For this review, take the finished solid that the model builds, in its own axes (mm). Face numbers are marked on the shaded views. A direction names the side the tool comes from. Give positions to 0.01 mm unless a question says otherwise; leave off trailing zeros. Write each loop counter-clockwise with the first axis right and the second up, starting at its lowest first coordinate (ties: lowest second). Pieces come first, ordered by that corner, then holes.
Q1. Machinability: for the marked faces 4, 5, 6 and 7, which of the approach directions +Z, -Z, +X, -X, +Y, -Y give a long, thin tool a straight path to every point of the face, cutting with its end or side? Answer none if there is none.
Q2. For line 1 (Z direction, x = 0, y = 9.75); line 2 (Z direction, x = 0.5, y = 4.75); line 3 (X direction, y = 13, z = -5), list the stretches that pass through material, from the lowest coordinate up.
Q3. We need section A-A (y = 5.5). Write out the cut boundary in (x, z) (1 decimal).
Q4. Mouldability with a two-part tool opening along Y and no side actions: class the marked faces 1, 2 and 3 as released by +Y, released by -Y, zero draft, split by the parting line, or undercut.
Q5. We need section B-B (z = -10). Give the number of separate pieces and of enclosed holes in the cut face, then the cut area to 3 significant figures.
Q6. Insertion check: P1, Ø1, axis at y = 9.5, z = -12.5, coming from the +X side; P2, Ø1, axis at x = -4, y = 8, coming from the +Z side; P3, Ø3, axis at y = 8, z = -14, coming from the +X side. Each pin has a flat end and moves straight along its axis. Give the tip position at first contact, or say it passes through.
```python
from build123d import *

# Parameters (mm, degrees)
CUT_EXTRUDE2_DEPTH       = 15.16264375
SKETCH5_W                = 4.35
SKETCH5_H                = 6.35
SKETCH6_R                = 1.5875
BOSS_EXTRUDE2_DEPTH      = 1
BOSS_EXTRUDE2_DEPTH_BACK = 9.525


with BuildPart() as part:
    # Sketch2 → Revolve-Thin1 (revolve)
    with BuildSketch(Plane.XY):
        Polygon((-24.60625, 0), (-24.293567435, 1.166947221), (-22.00484761, 1.166947221), (-21.79908333, 2.333894442), (-15.936399675, 3.36764375), (-15.203164833, 4.63764375), (-13.6921875, 4.63764375), (-13.6921875, 14.16264375), (0, 14.16264375), (0, 13.96420625), (-13.49375, 13.96420625), (-13.49375, 4.43920625), (-15.088596889, 4.43920625), (-15.810814222, 3.188289135), (-21.62778851, 2.162599622), (-21.838338777, 0.968509721), (-24.141300985, 0.968509721), (-24.414574094, -0.051359404), align=None)
    revolve(axis=Axis((0, 0, 0), (0, 1, 0)))

    # Sketch4 → Cut-Extrude2 (cut, through all)
    with BuildSketch(Plane(origin=(0, 0, 0), x_dir=(1, 0, 0), z_dir=(0, 1, 0))):
        with BuildLine():
            ThreePointArc((-18.702022535, -7.864281481), (-14.345950127, -14.345950127), (-7.864281481, -18.702022535))
            ThreePointArc((-7.864281481, -18.702022535), (-4.937265584, -17.507944491), (-6.131343629, -14.580928594))
            ThreePointArc((-6.131343629, -14.580928594), (-11.184740796, -11.184740796), (-14.580928594, -6.131343629))
            ThreePointArc((-14.580928594, -6.131343629), (-17.507944491, -4.937265584), (-18.702022535, -7.864281481))
        make_face()
        with BuildLine():
            ThreePointArc((-7.864281481, 18.702022535), (-14.345950127, 14.345950127), (-18.702022535, 7.864281481))
            ThreePointArc((-18.702022535, 7.864281481), (-17.507944491, 4.937265584), (-14.580928594, 6.131343629))
            ThreePointArc((-14.580928594, 6.131343629), (-11.184740796, 11.184740796), (-6.131343629, 14.580928594))
            ThreePointArc((-6.131343629, 14.580928594), (-4.937265584, 17.507944491), (-7.864281481, 18.702022535))
        make_face()
        with BuildLine():
            ThreePointArc((18.702022535, 7.864281481), (14.345950127, 14.345950127), (7.864281481, 18.702022535))
            ThreePointArc((7.864281481, 18.702022535), (4.937265584, 17.507944491), (6.131343629, 14.580928594))
            ThreePointArc((6.131343629, 14.580928594), (11.184740796, 11.184740796), (14.580928594, 6.131343629))
            ThreePointArc((14.580928594, 6.131343629), (17.507944491, 4.937265584), (18.702022535, 7.864281481))
        make_face()
        with BuildLine():
            ThreePointArc((7.864281481, -18.702022535), (14.345950127, -14.345950127), (18.702022535, -7.864281481))
            ThreePointArc((18.702022535, -7.864281481), (17.507944491, -4.937265584), (14.580928594, -6.131343629))
            ThreePointArc((14.580928594, -6.131343629), (11.184740796, -11.184740796), (6.131343629, -14.580928594))
            ThreePointArc((6.131343629, -14.580928594), (4.937265584, -17.507944491), (7.864281481, -18.702022535))
        make_face()
    extrude(amount=CUT_EXTRUDE2_DEPTH, mode=Mode.SUBTRACT)

    # Sketch5 → Revolve1 (revolve)
    with BuildSketch(Plane.XY):
        with Locations((-15.8671875, 9.40014375)):
            Rectangle(SKETCH5_W, SKETCH5_H)
    revolve(axis=Axis((0, 0, 0), (0, 1, 0)))

    # Sketch6 → Boss-Extrude2 (add, two sides)
    with BuildSketch(Plane.XZ.offset(-4.43920625)) as boss_extrude2_sk:
        Circle(SKETCH6_R)
    extrude(amount=BOSS_EXTRUDE2_DEPTH)
    extrude(boss_extrude2_sk.sketch, amount=-BOSS_EXTRUDE2_DEPTH_BACK)


solid = part.part
```
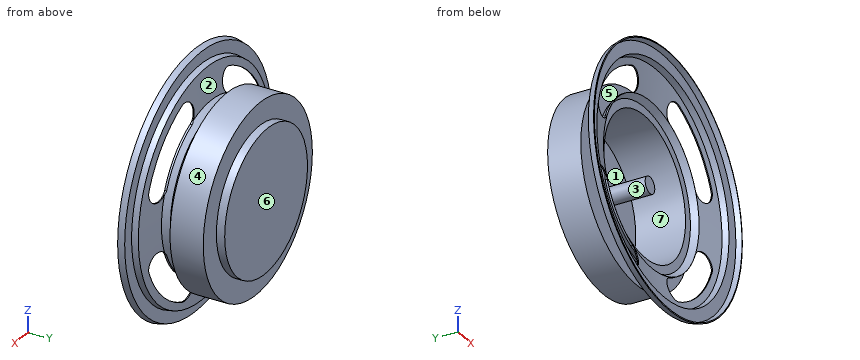
Computed:
1. face 4: +Y
1. face 5: none
1. face 6: +Z, -Z, +X, -X, +Y
1. face 7: -Y
2. line 1: z = -18.04 to -13.49, -1.59 to 1.59, 13.49 to 18.04
2. line 2: z = -13.68 to -13.48, -1.51 to 1.51, 13.48 to 13.68
2. line 3: x = -12.75 to -12.53, 12.53 to 12.75
3. outline: circle Ø27.4 at (0, 0); circle Ø3.2 at (0, 0); hole circle Ø27 at (0, 0)
4. face 1: released by -Y
4. face 2: undercut
4. face 3: zero draft
5. separate pieces: 3
5. enclosed holes: 0
5. area: 85.4 mm2
6. P1: stops at x = 13.47
6. P2: stops at z = 17.7
6. P3: stops at x = 13.01
